The model under review builds one solid part; all positions refer to its coordinate system, in mm. A direction names the side the tool comes from. Round coordinates to 2 decimals unless told otherwise and drop trailing zeros. Order: outer loops, then holes, each group sorted by start corner. A loop starts at its lowest first (then second) coordinate and runs counter-clockwise, first axis right, second up.
```python
from build123d import *

# Parameters (mm, degrees)
F0_W     = 8.7084230036
F0_H     = 38.9699079096
F2_W     = 90.2628563344
F2_H     = 34.500811249
F3_DEPTH = 6.75614


with BuildPart() as f1:
    # F0 (on Front) → F1 (revolve)
    with BuildSketch(Plane.XZ):
        with Locations((-4.3542115018, 19.4849539548)):
            Rectangle(F0_W, F0_H)
    revolve(axis=Axis((0, 0, 19.4849539548), (0, 0, 1)))

    # F2 (on Top) → F3 (join)
    with BuildSketch(Plane.XY):
        with Locations((13.2931489497, 0)):
            Rectangle(F2_W, F2_H)
    extrude(amount=-F3_DEPTH)


solid = f1.part
```
(1) Consider section A-A (x = 0). Write out the cut boundary in (y, z).
Data:
outline: (-17.25, -6.76) - (17.25, -6.76) - (17.25, 0) - (8.71, 0) - (8.71, 38.97) - (-8.71, 38.97) - (-8.71, 0) - (-17.25, 0) - close
(2) Insertion check: pin 1 (1.5 mm diameter, centred on y = -6.5, z = 18.5, fed in from -X); pin 2 (3 mm diameter, centred on x = 12.5, y = 12, fed in from +Z); pin 3 (3 mm diameter, centred on x = 3, z = 0.5, fed in from +Y); pin 4 (12 mm diameter, centred on y = -13.5, z = 31.5, fed in from +X). Each pin has a flat end and moves straight along its axis. Give the tip position at first contact, or say it passes through.
Data:
pin 1: stops at x = -6.54
pin 2: stops at z = 0
pin 3: stops at y = 17.25
pin 4: stops at x = 4.43
(3) To check wall thickness, follow probe 1 along Z at (x, y) = (26, -6.5); probe 2 along X at (y, z) = (4, 19); probe 3 along X at (y, z) = (6, 5.5). State the ranges of each line that lie inside material, in increasing order.
Data:
probe 1: z = -6.76 to 0
probe 2: x = -7.74 to 7.74
probe 3: x = -6.31 to 6.31
(4) Consider section B-B (y = 0). Write out the cut boundary in (x, z).
Data:
outline: (-31.84, -6.76) - (58.42, -6.76) - (58.42, 0) - (8.71, 0) - (8.71, 38.97) - (-8.71, 38.97) - (-8.71, 0) - (-31.84, 0) - close
(5) Consider section C-C (z = 27). Write out the cut boundary in (x, y), and give its area (3 significant figures).
Data:
outline: circle Ø17.42 at (0, 0)
area: 238 mm2
(6) For faces 1 (the cylindrical face through (-4.682, -7.343, 19.758)), 2 (the flat face through (13, 17.25, -3)), list the 3-axis set-ups (+Z, -Z, +X, -X, +Y, -Y) from which the entire face can be reached by the end or side of a thin tool; tool diameter is ignored.
Data:
face 1: +Z
face 2: +Z, -Z, +X, -X, +Y
(7) Consider section D-D (x = 10.5). Write out the cut boundary in (y, z).
Data:
outline: (-17.25, -6.76) - (17.25, -6.76) - (17.25, 0) - (-17.25, 0) - close
